The model under review builds one solid part; all positions refer to its coordinate system, in mm. A direction names the side the tool comes from. Round coordinates to 2 decimals unless told otherwise and drop trailing zeros. Order: outer loops, then holes, each group sorted by start corner. A loop starts at its lowest first (then second) coordinate and runs counter-clockwise, first axis right, second up. Notation, with made-up numbers: M 2.25,52 L 40.25,52 A7 cw 40.25,56 Z; hole C -27,45.25 d4. An arc over 180 degrees is marked long. Answer as a JSON object with one key per item and string values. Group by question number.
1. Add section A-A on y = -9. State the section outline as (x, z) points.
2. Clearance check with flat-ended pins moving along their axes: P1, Ø12.5, axis at x = 23, y = -112, coming from the +Z side; P2, Ø6, axis at x = 2.5, z = 17.5, coming from the +Y side; P3, Ø5, axis at x = 10.5, z = 37, coming from the -Y side; P4, Ø3, axis at x = 11, z = 2.5, coming from the -Y side. State where each tip first meets the part, or that it passes through.
3. Add section B-B on z = 21.5. State the section outline as (x, y) points, and give its area (3 significant figures).
4. Machinability: for faces 1 (the face through (49.73, -96.85, 28.65)), 2 (the face through (29.662, -103.685, 2.028)), 3 (the face through (44.156, -30, 2)), 4 (the face through (-7.312, -123.826, 52.496)), which of the approach directions +Z, -Z, +X, -X, +Y, -Y give a long, thin tool a straight path to every point of the face, cutting with its end or side? Answer none if there is none.
5. Mouldability with a two-part tool opening along Y and no side actions: class faces 5 (the face through (48, -100.3, 52.6)), 6 (the face through (57.51, -77.16, 29.35)), 7 (the face through (52.042, -88.179, 28.65)) as released by +Y, released by -Y, zero draft, split by the parting line, or undercut.
6. To check wall thickness, follow probe 1 along X at (y, z) = (-100.5, 22.5); probe 2 along X at (y, z) = (-90.5, 19); probe 3 along Z at (x, y) = (33, -84.5). State the ranges of each line that lie inside material, in increasing order. Write a range as [from, to].
7. Add section C-C on z = 30.5. State the section outline as (x, y) points.
```python
from build123d import *

# Parameters (mm, degrees)
F1_DEPTH  = 4
F2_R      = 5
F4_DEPTH  = 50
F6_DEPTH  = 25
F7_R      = 5
F8_R      = 2
F10_DEPTH = 25
F12_DEPTH = 25
F14_DEPTH = 25
F15_R     = 5


with BuildPart() as f1:
    # F0 (on Top) → F1 (new body)
    with BuildSketch(Plane.XY):
        with BuildLine():
            Line((49.8126317561, 22.0112954478), (-40.1873682439, 22.0112954478))
            ThreePointArc((-40.1873682439, 22.0112954478), (-47.2584360558, 19.0823632597), (-50.1873682439, 12.0112954478))
            Line((-50.1873682439, 12.0112954478), (-50.1873682439, -97.9887045522))
            Line((-50.1873682439, -97.9887045522), (-33.0722484738, -97.9887045522))
            Line((-33.0722484738, -97.9887045522), (59.8126317561, -97.9887045522))
            Line((59.8126317561, -97.9887045522), (59.8126317561, 12.0112954478))
            ThreePointArc((59.8126317561, 12.0112954478), (56.8836995679, 19.0823632597), (49.8126317561, 22.0112954478))
        make_face()
        with BuildLine():
            Line((-34.0809039772, -59.2981277779), (-34.0809039772, -2.0396176167))
            ThreePointArc((-34.0809039772, -2.0396176167), (-32.6164378831, 1.4959162892), (-29.0809039772, 2.9603823833))
            Line((-29.0809039772, 2.9603823833), (39.1555567086, 2.9603823833))
            ThreePointArc((39.1555567086, 2.9603823833), (42.6910906145, 1.4959162892), (44.1555567086, -2.0396176167))
            Line((44.1555567086, -2.0396176167), (44.1555567086, -59.2981277779))
            ThreePointArc((44.1555567086, -59.2981277779), (42.6910906145, -62.8336616838), (39.1555567086, -64.2981277779))
            Line((39.1555567086, -64.2981277779), (-29.0809039772, -64.2981277779))
            ThreePointArc((-29.0809039772, -64.2981277779), (-32.6164378831, -62.8336616838), (-34.0809039772, -59.2981277779))
        make_face(mode=Mode.SUBTRACT)
        Polygon((-18.8066744284, -131.4782482004), (59.8126317561, -97.9887045522), (-33.0722484738, -97.9887045522), align=None)
    extrude(amount=F1_DEPTH)

    # F2
    f2_edges = [f1.edges().sort_by_distance(p)[0] for p in [
        (-33.072248, -97.988705, 2),
        (-50.187368, -97.988705, 2),
        (59.812632, -97.988705, 2),
        (-18.806674, -131.478248, 2),
    ]]
    fillet(f2_edges, radius=F2_R)

    # F3 (on face) → F4 (join)
    with BuildSketch(Plane.XY.offset(4)):
        with BuildLine():
            Line((-6.9660247439, -120.9997456811), (-16.1661150585, -124.9187172558))
            Line((-16.1661150585, -124.9187172558), (-21.6526752631, -112.0385908154))
            Line((-21.6526752631, -112.0385908154), (49.3260715515, -81.8037038021))
            Line((49.3260715515, -81.8037038021), (54.8126317561, -94.6838302426))
            Line((54.8126317561, -94.6838302426), (45.6125414415, -98.6028018173))
            Line((45.6125414415, -98.6028018173), (47.5720272288, -103.2028469746))
            Line((47.5720272288, -103.2028469746), (56.7721175434, -99.2838753999))
            ThreePointArc((56.7721175434, -99.2838753999), (58.9838083848, -97.4408731388), (59.8126317561, -94.6838302426))
            Line((59.8126317561, -94.6838302426), (59.8126317561, -73.8051433371))
            Line((59.8126317561, -73.8051433371), (5.2046610063, -97.0665546714))
            Line((5.2046610063, -97.0665546714), (1.9289534576, -98.4619110571))
            Line((1.9289534576, -98.4619110571), (-23.9415310778, -109.4819869532))
            Line((-23.9415310778, -109.4819869532), (-27.5260314097, -111.0088801064))
            Line((-27.5260314097, -111.0088801064), (-20.7661602158, -126.8782030431))
            ThreePointArc((-20.7661602158, -126.8782030431), (-18.0332724951, -129.5570060682), (-14.2066292711, -129.5187624131))
            Line((-14.2066292711, -129.5187624131), (-5.0065389565, -125.5997908384))
            Line((-5.0065389565, -125.5997908384), (-6.9660247439, -120.9997456811))
        make_face()
        Polygon((-31.7770776261, -101.0292187648), (-27.5260314097, -111.0088801064), (-23.9415310778, -109.4819869532), (-46.2875531446, -57.0229636434), (-49.8720534765, -58.5498567966), align=None)
        Polygon((1.9289534576, -98.4619110571), (5.2046610063, -97.0665546714), (-8.3174404532, -65.3223706937), (-11.5931480018, -66.7177270794), align=None)
    extrude(amount=F4_DEPTH)

    # F5 (on face) → F6 (cut)
    with BuildSketch(Plane.XY.offset(4)):
        Polygon((10.3267065007, -119.0682730989), (21.2827441361, -114.4013189065), (16.1116256489, -102.2617164104), (5.1555880134, -106.9286706028), align=None)
        Polygon((16.1116256489, -102.2617164104), (21.2827441361, -114.4013189065), (32.2387817716, -109.734364714), (27.0676632843, -97.5947622179), align=None)
    extrude(amount=-F6_DEPTH, mode=Mode.SUBTRACT)

    # F7
    f7_edges = [f1.edges().sort_by_distance(p)[0] for p in [
        (-5.986282, -123.299768, 54),
        (46.592284, -100.902824, 54),
        (46.592284, -100.902824, 4),
        (-5.986282, -123.299768, 4),
        (32.238782, -109.734365, 2),
        (10.326707, -119.068273, 2),
        (27.067663, -97.594762, 2),
        (5.155588, -106.928671, 2),
    ]]
    fillet(f7_edges, radius=F7_R)

    # F8
    f8_edges = [f1.edges().sort_by_distance(p)[0] for p in [
        (49.326072, -81.803704, 29),
        (54.812632, -94.68383, 29),
        (-21.652675, -112.038591, 29),
        (-16.166115, -124.918717, 29),
    ]]
    fillet(f8_edges, radius=F8_R)

    # F9 (on face) → F10 (cut)
    with BuildSketch(Plane(origin=(-59.7381223873, -25.4467071035, 0), x_dir=(-0.3918971575, 0.9200090315, 0), z_dir=(0.9200090315, 0.3918971575, 0))):
        Polygon((-34.321681049, 54), (-91.3417988043, 54), (-34.321681049, 4), align=None)
    extrude(amount=-F10_DEPTH, mode=Mode.SUBTRACT)

    # F11 (on face) → F12 (cut)
    with BuildSketch(Plane.XY.offset(4)):
        with BuildLine():
            ThreePointArc((-36.3771227834, -97.9887045522), (-33.6200798872, -98.8175279234), (-31.7770776261, -101.0292187648))
            Line((-31.7770776261, -101.0292187648), (-49.8720534765, -58.5498567966))
            Line((-49.8720534765, -58.5498567966), (-50.1873682439, -57.809630877))
            Line((-50.1873682439, -57.809630877), (-50.1873682439, -92.9887045522))
            ThreePointArc((-50.1873682439, -92.9887045522), (-48.7229021499, -96.5242384581), (-45.1873682439, -97.9887045522))
            Line((-45.1873682439, -97.9887045522), (-36.3771227834, -97.9887045522))
        make_face()
    extrude(amount=-F12_DEPTH, mode=Mode.SUBTRACT)

    # F13 (on face) → F14 (cut)
    with BuildSketch(Plane(origin=(-30.5919303032, -13.0312748216, 0), x_dir=(-0.3918971575, 0.9200090315, 0), z_dir=(0.9200090315, 0.3918971575, 0))):
        Polygon((-56.8375897235, 54), (-91.3417988043, 54), (-56.8375897235, 4), align=None)
    extrude(amount=-F14_DEPTH, mode=Mode.SUBTRACT)

    # F15
    f15_edges = [f1.edges().sort_by_distance(p)[0] for p in [
        (59.812632, -73.805143, 29),
    ]]
    fillet(f15_edges, radius=F15_R)


solid = f1.part
```
Recorded:
{
 "1": {"outline": "M -50.19,0 L -34.08,0 L -34.08,4 L -50.19,4 Z; M 44.16,0 L 59.81,0 L 59.81,4 L 44.16,4 Z"},
 "2": {"P1": "passes through", "P2": "stops at y = -83.67", "P3": "stops at y = -99.41", "P4": "stops at y = -105.09"},
 "3": {"outline": "M -42.05,-76.91 L -20.77,-126.88 A5 ccw -14.21,-129.52 L -5.01,-125.6 L -6.97,-121 L -14.33,-124.13 A2 cw -16.95,-123.08 L -20.87,-113.88 A2 cw -19.81,-111.25 L 47.49,-82.59 A2 cw 50.11,-83.64 L 54.03,-92.84 A2 cw 52.97,-95.47 L 45.61,-98.6 L 47.57,-103.2 L 56.77,-99.28 A5 ccw 59.81,-94.68 L 59.81,-81.37 A5 ccw 52.85,-76.77 L 5.2,-97.07 L -3.58,-76.43 L -6.86,-77.83 L 1.93,-98.46 L -23.94,-109.48 L -38.47,-75.38 Z", "area": "848 mm²"},
 "4": {"face 1": "+Z", "face 2": "+Z, -Z, -Y", "face 3": "+Z, -Z", "face 4": "+Z, +X"},
 "5": {"face 5": "released by -Y", "face 6": "released by +Y", "face 7": "undercut"},
 "6": {"probe 1": "x = [-32, -27.77], [-2.86, 5.44], [46.42, 53.92]", "probe 2": "x = [-36.26, -32.03], [-1.46, 2.41], [20.62, 28.91], [53.03, 59.81]", "probe 3": "z = [0, 4]"},
 "7": {"outline": "M -38.03,-86.35 L -20.77,-126.88 A5 ccw -14.21,-129.52 L -5.01,-125.6 L -6.97,-121 L -14.33,-124.13 A2 cw -16.95,-123.08 L -20.87,-113.88 A2 cw -19.81,-111.25 L 47.49,-82.59 A2 cw 50.11,-83.64 L 54.03,-92.84 A2 cw 52.97,-95.47 L 45.61,-98.6 L 47.57,-103.2 L 56.77,-99.28 A5 ccw 59.81,-94.68 L 59.81,-81.37 A5 ccw 52.85,-76.77 L 5.2,-97.07 L -1.15,-82.15 L -4.43,-83.54 L 1.93,-98.46 L -23.94,-109.48 L -34.44,-84.83 Z"}
}
